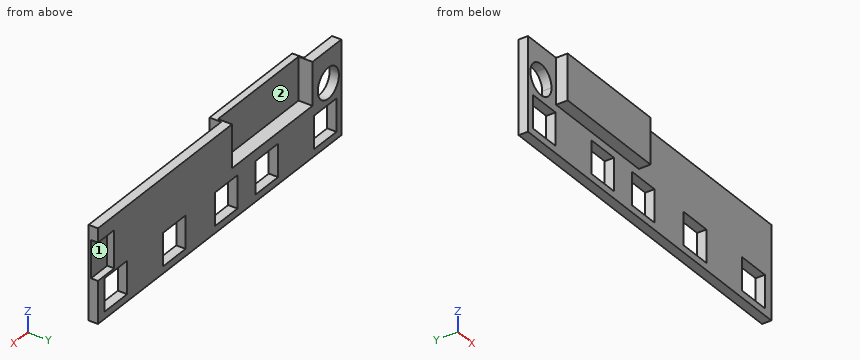
```python
from build123d import *

# Parameters (mm, degrees)
F0_W     = 40.8479798585
F0_H     = 4
F0_W_2   = 7
F0_H_2   = 7
F1_DEPTH = 2
F0_W_3   = 25.5042742938
F0_H_3   = 5.8133912664
F2_DEPTH = 4.5
F4_W     = 5
F4_H     = 8
F5_DEPTH = 1.5
F6_W     = 24.8026130721
F6_H     = 9.2125886586
F7_DEPTH = 3


with BuildPart() as f1:
    # F0 (on Front) → F1 (new body)
    with BuildSketch(Plane.XZ):
        with Locations((17.0760100707, 10)):
            Rectangle(F0_W, F0_H)
        with BuildLine():
            Line((-37.5, 12), (-37.5, 8))
            Line((-37.5, 8), (-34.75, 8))
            ThreePointArc((-34.75, 8), (-33.5, 8.25), (-32.25, 8))
            Line((-32.25, 8), (-28.8522541523, 8))
            Line((-28.8522541523, 8), (-28.8522541523, 12))
            Line((-28.8522541523, 12), (-37.5, 12))
        make_face()
        with BuildLine():
            Line((-37.5, 8), (-37.5, -8))
            Line((-37.5, -8), (37.5, -8))
            Line((37.5, -8), (37.5, 8))
            Line((37.5, 8), (-3.3479798585, 8))
            Line((-3.3479798585, 8), (-3.3479798585, 2.1866087336))
            Line((-3.3479798585, 2.1866087336), (-28.8522541523, 2.1866087336))
            Line((-28.8522541523, 2.1866087336), (-28.8522541523, 8))
            Line((-28.8522541523, 8), (-32.25, 8))
            ThreePointArc((-32.25, 8), (-30.7958365434, 6.8027756377), (-30.25, 5))
            ThreePointArc((-30.25, 5), (-35.3027756377, 2.2958365434), (-34.75, 8))
            Line((-34.75, 8), (-37.5, 8))
        make_face()
        with Locations((-32.5, -3)):
            Rectangle(F0_W_2, F0_H_2, mode=Mode.SUBTRACT)
        with Locations((-14.5, -3)):
            Rectangle(F0_W_2, F0_H_2, mode=Mode.SUBTRACT)
        with Locations((-2, -3)):
            Rectangle(F0_W_2, F0_H_2, mode=Mode.SUBTRACT)
        with Locations((14, -3)):
            Rectangle(F0_W_2, F0_H_2, mode=Mode.SUBTRACT)
        with Locations((32, -3)):
            Rectangle(F0_W_2, F0_H_2, mode=Mode.SUBTRACT)
    extrude(amount=F1_DEPTH)

    # F0 (on Front) → F2 (join)
    with BuildSketch(Plane.XZ):
        with Locations((-16.1001170054, 10)):
            Rectangle(F0_W_3, F0_H)
        with Locations((-16.1001170054, 5.0933043668)):
            Rectangle(F0_W_3, F0_H_3)
    extrude(amount=F2_DEPTH)

    # F4 (on face) → F5 (cut)
    with BuildSketch(Plane(origin=(0, 0, 0), x_dir=(-1, 0, 0), z_dir=(0, 1, 0))):
        with Locations((-35, 5)):
            Rectangle(F4_W, F4_H)
    extrude(amount=-F5_DEPTH, mode=Mode.SUBTRACT)

    # F6 (on face) → F7 (cut)
    with BuildSketch(Plane(origin=(0, 0, 0), x_dir=(-1, 0, 0), z_dir=(0, 1, 0))):
        with Locations((16.2086286582, 7.4240994873)):
            Rectangle(F6_W, F6_H)
    extrude(amount=-F7_DEPTH, mode=Mode.SUBTRACT)


solid = f1.part
```
Source: CAD feature listing. Evaluate the final solid. Frame: model axes, mm. Face numbers are marked on the shaded views. Give positions to 0.01 mm unless a question says otherwise; leave off trailing zeros. Loops run counter-clockwise (first coordinate to the right, second up) from the corner with the lowest first, then second, coordinate; pieces in that order, holes last. Notation, with made-up numbers: (40, 6) - (59, 6) arc R16 ccw to (59, 31) - close; hole circle Ø9 at (59, 40). An arc over 180 degrees is marked (long way). Use CSV: the item, a comma, the result in double quotes. Start each with the question number.
1. Section D-D (x = -20.5). Output: boundary loops of the cut face in (y, z), then the cut area to 3 significant figures.
2. Section B-B (z = -4.25). Output: boundary loops of the cut face in (x, y).
3. Ray query, L1, parallel to Z at x = -33.5, y = -0.95; L2, parallel to X at y = -1.1, z = 5; L3, parallel to X at y = -0.65, z = 10.5. Return the intervals inside material, ascending.
4. Draft query along Z for the marked faces 1 and 2. Return one class per face: +Z half, -Z half, draft (parallel to the pull), parting line (faces both ways), or undercut.
5. Section C-C (z = 3.5). Output: boundary loops of the cut face in (x, y).
6. Section A-A (x = -33.5). Output: boundary loops of the cut face in (y, z).
7. Pin query (flat end, axial travel): pin 1 (1 mm diameter, centred on x = -13.5, y = -1.5, fed in from +Z); pin 2 (2 mm diameter, centred on y = -3.5, z = 4.5, fed in from +X); pin 3 (1.5 mm diameter, centred on y = -3.5, z = 10, fed in from -X). Return the tip coordinate at first contact, or that it passes through.
Response:
1,outline,"(-4.5, 2.19) - (-2, 2.19) - (-2, -8) - (0, -8) - (0, 2.82) - (-3, 2.82) - (-3, 12) - (-4.5, 12) - close"
1,area,"37.0 mm²"
2,outline,"(-37.5, -2) - (-36, -2) - (-36, 0) - (-37.5, 0) - close; (-29, -2) - (-18, -2) - (-18, 0) - (-29, 0) - close; (-11, -2) - (-5.5, -2) - (-5.5, 0) - (-11, 0) - close; (1.5, -2) - (10.5, -2) - (10.5, 0) - (1.5, 0) - close; (17.5, -2) - (28.5, -2) - (28.5, 0) - (17.5, 0) - close; (35.5, -2) - (37.5, -2) - (37.5, 0) - (35.5, 0) - close"
3,L1,"-8 to -6.5, 0.5 to 1.75, 8.25 to 12"
3,L2,"-37.5 to -36.75, -30.25 to -28.61, -3.81 to 32.5"
3,L3,"-37.5 to -28.61, -3.81 to 37.5"
4,face 1,"undercut"
4,face 2,"draft"
5,outline,"(-37.5, -2) - (-36.38, -2) - (-36.38, 0) - (-37.5, 0) - close; (-30.62, -2) - (-28.85, -2) - (-28.85, -4.5) - (-3.35, -4.5) - (-3.35, -2) - (37.5, -2) - (37.5, -1.5) - (32.5, -1.5) - (32.5, 0) - (-3.81, 0) - (-3.81, -3) - (-28.61, -3) - (-28.61, 0) - (-30.62, 0) - close"
6,outline,"(-2, -8) - (0, -8) - (0, -6.5) - (-2, -6.5) - close; (-2, 0.5) - (0, 0.5) - (0, 1.75) - (-2, 1.75) - close; (-2, 8.25) - (0, 8.25) - (0, 12) - (-2, 12) - close"
7,pin 1,"z = 2.82"
7,pin 2,"x = -3.35"
7,pin 3,"x = -28.85"
